Could you check a few things on this drawing? It's one solid part, dimensions in mm from its lowest x, y, z. A direction names the side the tool comes from. Round coordinates to 2 decimals unless told otherwise and drop trailing zeros. Order: outer loops, then holes, each group sorted by start corner. A loop starts at its lowest first (then second) coordinate and runs counter-clockwise, first axis right, second up. Notation, with made-up numbers: (65.25, 88) -> (104.25, 88) arc R3 cw to (104.25, 92) -> close; hole circle Ø6 at (79.25, 16.25). An arc over 180 degrees is marked (long way). Use a Markdown table: item, result. Add a question column.
(1) On a 3-axis mill with a long thin cutter (end or side, diameter ignored), from which of +Z, -Z, +X, -X, +Y, -Y can I reach the whole of each face in a straight line? I mean the marked faces 1 and 2. Say none if no direction works.
(2) I'm going to push flat-ended pins straight in: P1, Ø3, axis at x = 18, y = 37, coming from the +Z side; P2, Ø3, axis at x = 16.5, z = 10, coming from the -Y side; P3, Ø3, axis at x = 12, z = 9.5, coming from the +Y side; P4, Ø1.6, axis at y = 21, z = 0.5, coming from the -X side. Where does each tip first touch, or does it pass through?
(3) I want a section at B-B, the plane z = 10. Please give me the cut outline in (x, y).
(4) If I drill on probe 1 along Z at (x, y) = (5.5, 9.5); probe 2 along Y at (x, z) = (9.5, 8.25); probe 3 along Z at (x, y) = (2, 9), over which ranges is the centre line in solid material (lowest first)?
(5) I want a section at C-C, the plane y = 35. Please give me the cut outline in (x, z).
(6) I want a section at A-A, the plane x = 16.5. Please give me the cut outline in (y, z), then the cut area to 3 significant figures.
(7) I want a section at D-D, the plane x = 22. Please give me the cut outline in (y, z).
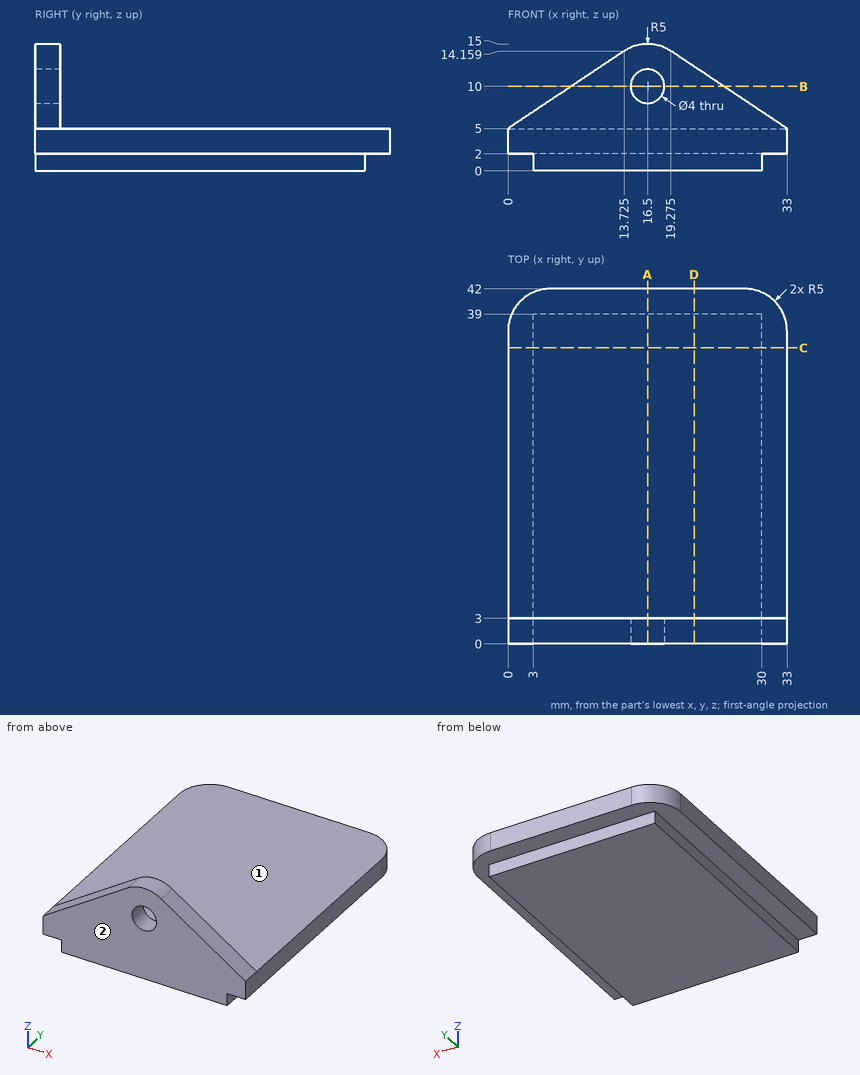
Taken from the geometry:
| question | item | result |
|---|---|---|
| 1 | face 1 | +Z, +X, -X, +Y |
| 1 | face 2 | +Z, -Z, +X, -X, -Y |
| 2 | P1 | stops at z = 5 |
| 2 | P2 | passes through |
| 2 | P3 | stops at y = 3 |
| 2 | P4 | stops at x = 3 |
| 3 | outline | (7.49, 0) -> (14.5, 0) -> (14.5, 3) -> (7.49, 3) -> close; (18.5, 0) -> (25.51, 0) -> (25.51, 3) -> (18.5, 3) -> close |
| 4 | probe 1 | z = 0 to 5 |
| 4 | probe 2 | y = 0 to 3 |
| 4 | probe 3 | z = 2 to 5 |
| 5 | outline | (0, 2) -> (3, 2) -> (3, 0) -> (30, 0) -> (30, 2) -> (33, 2) -> (33, 5) -> (0, 5) -> close |
| 6 | outline | (0, 0) -> (39, 0) -> (39, 2) -> (42, 2) -> (42, 5) -> (3, 5) -> (3, 8) -> (0, 8) -> close; (0, 12) -> (3, 12) -> (3, 15) -> (0, 15) -> close |
| 6 | area | 222 mm2 |
| 7 | outline | (0, 0) -> (39, 0) -> (39, 2) -> (42, 2) -> (42, 5) -> (3, 5) -> (3, 12.34) -> (0, 12.34) -> close |
